Read the model definition and answer for the solid it produces. Units are mm, in the model's axes. Give positions to 0.01 mm unless a question says otherwise; leave off trailing zeros. Write each loop counter-clockwise with the first axis right and the second up, starting at its lowest first coordinate (ties: lowest second). Pieces come first, ordered by that corner, then holes. Notation, with made-up numbers: M 52,46.5 L 100,46.5 A10 cw 100,54.5 Z; hole C 5,2 d6. An arc over 180 degrees is marked long. Use a Markdown table: item, result. Add a question column.
Item 1: Consider probe 1 along Y at (x, z) = (-1.3, 7.5); probe 2 along Z at (x, y) = (0.75, 110.5). Determine where each line is inside the solid, lowest interval first. Write a range as [from, to].
Item 2: A cutting plane is placed at A-A on x = -0.4. Determine the outline of the cut face in (y, z), then the cut area to 3 significant figures.
Item 3: A cutting plane is placed at B-B on z = -35. Determine the outline of the cut face in (x, y).
Autodesk Inventor part; units mm, degrees
ref_plane "YZ Plane" through (0, 0, 0) normal (1, 0, 0) x (0, 1, 0)
ref_plane "XZ Plane" through (0, 0, 0) normal (0, 1, 0) x (-1, 0, 0)
ref_plane "XY Plane" through (0, 0, 0) normal (0, 0, 1) x (1, 0, 0)
sketch "Skizze1" plane through (0, 0, 0) normal (1, 0, 0) x (0, 1, 0)
  line L0 (-176.4, 0) -> (176.4, 0)
  line L1 (0, -176.4) -> (0, 176.4)
  line L2 (126, 126) -> (-126, 126)
  line L3 (-126, 126) -> (-126, -126)
  line L4 (-126, -126) -> (126, -126)
  line L5 (126, -126) -> (126, 126)
  line L6 (111, 111) -> (-111, 111)
  line L7 (-111, 111) -> (-111, -111)
  line L8 (-111, -111) -> (111, -111)
  line L9 (111, -111) -> (111, 111)
  point P0 (0, 0)
  dimension "d0" = 252
  dimension "d1" = 252
  dimension "d2" = 222
  dimension "d3" = 222
extrude "Extrusion1" add sketch "Skizze1" along normal mid plane 3 contours L3 L2 L1 L6 L7 L0 | L0 L7 L8 L1 L4 L3 | L2 L5 L0 L9 L6 L1 | L1 L8 L9 L0 L5 L4
fillet "Rundung1" radius 3 4 edges at (0, 126, 126) (0, 126, -126) (0, -126, -126) (0, -126, 126)
fillet "Rundung2" radius 3 4 edges at (0, -111, -111) (0, 111, -111) (0, 111, 111) (0, -111, 111)
properties part number "Frontplatte" material "Stahl"
Filled in:
| question | item | result |
|---|---|---|
| 1 | probe 1 | [-126, -111], [111, 126] |
| 1 | probe 2 | [-126, -109.66], [109.66, 126] |
| 2 | outline | M -126,-123 A3 ccw -123,-126 L 123,-126 A3 ccw 126,-123 L 126,123 A3 ccw 123,126 L -123,126 A3 ccw -126,123 Z; hole M -111,-108 A3 ccw -108,-111 L 108,-111 A3 ccw 111,-108 L 111,108 A3 ccw 108,111 L -108,111 A3 ccw -111,108 Z |
| 2 | area | 14,200 mm² |
| 3 | outline | M -1.5,-126 L 1.5,-126 L 1.5,-111 L -1.5,-111 Z; M -1.5,111 L 1.5,111 L 1.5,126 L -1.5,126 Z |
